Read the model definition and answer for the solid it produces. Units are mm, in the model's axes. A direction names the side the tool comes from. Coordinates: 2 decimals unless noted, no trailing zeros. Write each loop counter-clockwise with the first axis right and the second up, starting at its lowest first coordinate (ties: lowest second). Pieces come first, ordered by that corner, then holes.
Item 1: Straight lines are drawn through the part: probe 1 along Z at (x, y) = (-18.5, 0.5); probe 2 along Y at (x, z) = (20, 10); probe 3 along Z at (x, y) = (4, 3.75). For each, find the intervals that lie inside material, in ascending order.
Item 2: Section B-B (z = 0) is taken. Give the vertices of the cut face in (x, y).
Item 3: Section A-A (x = -10) is taken. Give the vertices of the cut face in (y, z).
Item 4: Section D-D (z = 9) is taken. Give the vertices of the cut face in (x, y), then the cut area to 3 significant figures.
Item 5: Each of these flat-tipped pins is pushed along its axis until it touches: P1, Ø16.5, axis at x = -5, z = -4, coming from the -Y side; P2, Ø0.9, axis at x = 2, y = 5, coming from the -Z side; P3, Ø2, axis at x = -10.5, y = 8, coming from the +Z side; P4, Ø1, axis at x = 21.27, z = 8.79, coming from the -Y side. Where does it stop, or does it pass through?
Item 6: Section C-C (y = 1.5) is taken. Give the vertices of the cut face in (x, z).
Item 7: A tool of negligible diameter and unlimited length cuts with its end or side. For faces 1 (the face through (0, 0, 20)), 2 (the face through (0, 4, -9.144)), 3 (the face through (7.38, 4.23, -6.97)), 4 (the face through (0, -2, 7.366)), from which of +Z, -Z, +X, -X, +Y, -Y can it reach the whole face along a straight path? Write none if from no direction.
Item 8: Determine the mould class of faces 5 (the face through (0, -2, 30.226)), 6 (the face through (21.8, 1.4, 8.2)), 7 (the face through (4.953, -2, 19)) for opening direction X: released by +X, released by -X, zero draft, split by the parting line, or undercut.
from build123d import *

# Parameters (mm, degrees)
SKETCH1_W           = 45.2755
SKETCH1_H           = 20.32
BOSS_EXTRUDE1_DEPTH = 2.794
SKETCH2_R           = 7.9375
BOSS_EXTRUDE2_DEPTH = 12.0015
BOSS_EXTRUDE3_DEPTH = 2.921
SKETCH5_W           = 9.906
SKETCH5_H           = 20.066
SKETCH5_H_2         = 2.794
BOSS_EXTRUDE4_DEPTH = 3.302
SKETCH6_R           = 0.79375
CUT_EXTRUDE1_DEPTH  = 40.624674173


with BuildPart() as part:
    # Sketch1 → Boss-Extrude1 (new body)
    with BuildSketch(Plane(origin=(0, 0, 0), x_dir=(1, 0, 0), z_dir=(0, 1, 0))):
        Rectangle(SKETCH1_W, SKETCH1_H)
    extrude(amount=BOSS_EXTRUDE1_DEPTH)

    # Sketch2 → Boss-Extrude2 (add)
    with BuildSketch(Plane(origin=(0, 2.794, 0), x_dir=(1, 0, 0), z_dir=(0, 1, 0))):
        with Locations(Location((-12.92225, 0, 0), (0, 0, 270))):
            Circle(SKETCH2_R)
        with Locations(Location((12.92225, 0, 0), (0, 0, 90))):
            Circle(SKETCH2_R)
    extrude(amount=BOSS_EXTRUDE2_DEPTH)

    # Sketch3 → Boss-Extrude3 (add)
    with BuildSketch(Plane(origin=(0, 2.794, 0), x_dir=(1, 0, 0), z_dir=(0, 1, 0))):
        with BuildLine():
            Line((-5.156416146, 9.144), (5.156416146, 9.144))
            ThreePointArc((5.156416146, 9.144), (7.378916146, 6.9215), (5.156416146, 4.699))
            Line((5.156416146, 4.699), (-5.156416146, 4.699))
            ThreePointArc((-5.156416146, 4.699), (-7.378916146, 6.9215), (-5.156416146, 9.144))
        make_face()
    extrude(amount=BOSS_EXTRUDE3_DEPTH)

    # Sketch5 → Boss-Extrude4 (add)
    with BuildSketch(Plane.XZ):
        with Locations((0, 20.193)):
            Rectangle(SKETCH5_W, SKETCH5_H)
        with Locations((0, 8.763)):
            Rectangle(SKETCH5_W, SKETCH5_H_2)
    extrude(amount=BOSS_EXTRUDE4_DEPTH)

    # Sketch6 → Cut-Extrude1 (cut, through all)
    with BuildSketch(Plane(origin=(0, 2.794, 0), x_dir=(1, 0, 0), z_dir=(0, 1, 0))):
        with Locations(Location((-21.2725, 8.79475, 0), (0, 0, 270))):
            Circle(SKETCH6_R)
        with Locations(Location((-21.2725, -8.79475, 0), (0, 0, 270))):
            Circle(SKETCH6_R)
        with Locations(Location((21.2725, -8.79475, 0), (0, 0, 270))):
            Circle(SKETCH6_R)
        with Locations(Location((21.2725, 8.79475, 0), (0, 0, 270))):
            Circle(SKETCH6_R)
    extrude(amount=-CUT_EXTRUDE1_DEPTH, mode=Mode.SUBTRACT)


solid = part.part
Established:
1. probe 1: z = -10.16 to 10.16
1. probe 2: y = 0 to 2.79
1. probe 3: z = -9.14 to -4.7
2. outline: (-22.64, 0) - (22.64, 0) - (22.64, 2.79) - (20.86, 2.79) - (20.86, 14.8) - (4.98, 14.8) - (4.98, 2.79) - (-4.98, 2.79) - (-4.98, 14.8) - (-20.86, 14.8) - (-20.86, 2.79) - (-22.64, 2.79) - close
3. outline: (0, -10.16) - (2.79, -10.16) - (2.79, -7.38) - (14.8, -7.38) - (14.8, 7.38) - (2.79, 7.38) - (2.79, 10.16) - (0, 10.16) - close
4. outline: (-22.64, 0) - (-22.04, 0) - (-22.04, 2.79) - (-22.64, 2.79) - close; (-20.51, 0) - (-4.95, 0) - (-4.95, -3.3) - (4.95, -3.3) - (4.95, 0) - (20.51, 0) - (20.51, 2.79) - (-20.51, 2.79) - close; (22.04, 0) - (22.64, 0) - (22.64, 2.79) - (22.04, 2.79) - close
4. area: 151 mm2
5. P1: stops at y = 0
5. P2: stops at z = -9.14
5. P3: stops at z = 7.81
5. P4: passes through
6. outline: (-22.64, -10.16) - (22.64, -10.16) - (22.64, 10.16) - (-22.64, 10.16) - close; hole circle Ø1.59 at (-21.27, -8.79); hole circle Ø1.59 at (-21.27, 8.79); hole circle Ø1.59 at (21.27, -8.79); hole circle Ø1.59 at (21.27, 8.79)
7. face 1: +Z, +X, -X, +Y
7. face 2: -Z, +X, -X, +Y
7. face 3: +Y
7. face 4: -Z, +X, -X, -Y
8. face 5: zero draft
8. face 6: undercut
8. face 7: released by +X
